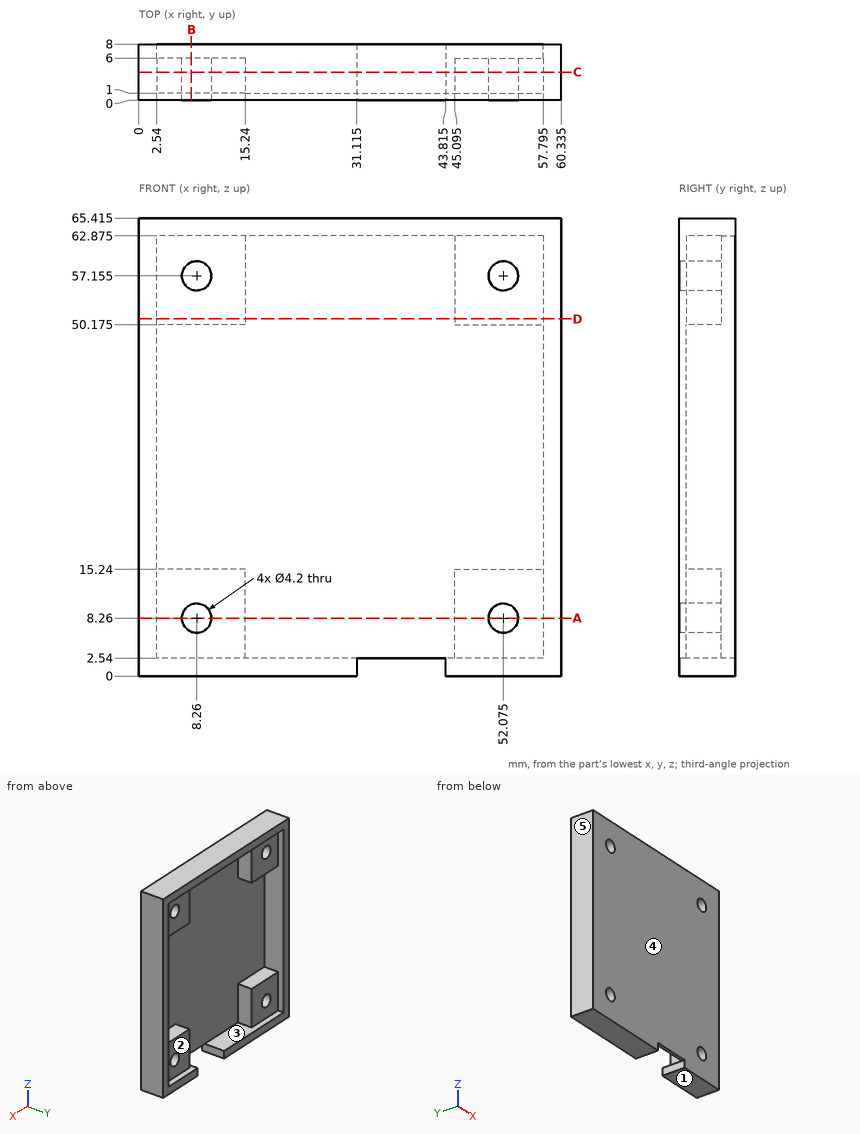
The figure shows three views and two pictorial views of one solid part (mm, origin at its lowest corner). Answer the questions. A direction names the side the tool comes from. Round coordinates to 2 decimals unless told otherwise and drop trailing zeros. Write each loop counter-clockwise with the first axis right and the second up, starting at its lowest first coordinate (ties: lowest second). Pieces come first, ordered by that corner, then holes. Notation, with made-up numbers: (-24.5, 6.5) - (9.5, 6.5) arc R20 ccw to (9.5, 37.5) - close; hole circle Ø3 at (58, -4). An arc over 180 degrees is marked (long way). Use one line per item in the form item = value. Start each with the question number.
Item 1: A cutting plane is placed at A-A (z = 8.26). Write down the section's boundary in (x, y) (3 decimals), plus the area to 3 significant figures.
Item 2: A cutting plane is placed at D-D (z = 51). Write down the section's boundary in (x, y) (3 decimals), plus the area to 3 significant figures.
Item 3: Determine the mould class of the marked faces 3, 4 and 5 for opening direction X: +X half, -X half, draft (parallel to the pull), parting line (faces both ways), or undercut.
Item 4: Flat-ended cylindrical pins translate along their axes: pin 1 Ø4 at (x, z) = (8.26, 57.155) entering from -Y; pin 2 Ø2 at (x, y) = (42.5, 6) entering from -Z (3 decimals); pin 3 Ø4 at (x, z) = (50, 12) entering from +Y. Find the tip coordinate at first contact, or state that the pin passes through.
Item 5: A tool of negligible diameter and unlimited length cuts with its end or side. For the marked faces 1 and 2, from which of +Z, -Z, +X, -X, +Y, -Y can it reach the whole face along a straight path? Write none if from no direction.
Item 6: A cutting plane is placed at C-C (y = 4). Write down the section's boundary in (x, z) (3 decimals), plus the area to 3 significant figures.
Item 7: A cutting plane is placed at B-B (x = 7.5). Write down the section's boundary in (y, z) (3 decimals), plus the area to 3 significant figures.
Item 8: Find the intervals of material crossed by line 1 (Z direction, x = 8.26, y = 3.4) (3 decimals); line 2 (X direction, y = 0.75, z = 8) (3 decimals); line 3 (Z direction, x = 4, y = 2.5) (3 decimals), in increasing order. Write a range as [from, to].
The answers:
q1.outline = (0, 0) - (6.16, 0) - (6.16, 6) - (2.54, 6) - (2.54, 8) - (0, 8) - close; (10.36, 0) - (49.975, 0) - (49.975, 6) - (45.095, 6) - (45.095, 1) - (15.24, 1) - (15.24, 6) - (10.36, 6) - close; (54.175, 0) - (60.335, 0) - (60.335, 8) - (57.795, 8) - (57.795, 6) - (54.175, 6) - close
q1.area = 172 mm^2
q2.outline = (0, 0) - (60.335, 0) - (60.335, 8) - (57.795, 8) - (57.795, 6) - (45.095, 6) - (45.095, 1) - (15.24, 1) - (15.24, 6) - (2.54, 6) - (2.54, 8) - (0, 8) - close
q2.area = 223 mm^2
q3.face_3 = undercut
q3.face_4 = draft
q3.face_5 = -X half
q4.pin_1 = through
q4.pin_2 = 62.875
q4.pin_3 = 6
q5.face_1 = -Z, +X, -X, +Y, -Y
q5.face_2 = +Y
q6.outline = (0, 0) - (31.115, 0) - (31.115, 2.54) - (15.24, 2.54) - (15.24, 15.24) - (2.54, 15.24) - (2.54, 50.175) - (15.24, 50.175) - (15.24, 62.875) - (45.095, 62.875) - (45.095, 50.175) - (57.795, 50.175) - (57.795, 15.24) - (45.095, 15.24) - (45.095, 2.54) - (43.815, 2.54) - (43.815, 0) - (60.335, 0) - (60.335, 65.415) - (0, 65.415) - close; hole circle Ø4.2 at (8.26, 8.26); hole circle Ø4.2 at (8.26, 57.155); hole circle Ø4.2 at (52.075, 8.26); hole circle Ø4.2 at (52.075, 57.155)
q6.area = 1,170 mm^2
q7.outline = (0, 0) - (8, 0) - (8, 2.54) - (6, 2.54) - (6, 6.302) - (0, 6.302) - close; (0, 10.218) - (6, 10.218) - (6, 15.24) - (1, 15.24) - (1, 50.175) - (6, 50.175) - (6, 55.197) - (0, 55.197) - close; (0, 59.113) - (6, 59.113) - (6, 62.875) - (8, 62.875) - (8, 65.415) - (0, 65.415) - close
q7.area = 181 mm^2
q8.line_1 = [0, 6.16], [10.36, 15.24], [50.175, 55.055], [59.255, 65.415]
q8.line_2 = [0, 6.176], [10.344, 49.991], [54.159, 60.335]
q8.line_3 = [0, 15.24], [50.175, 65.415]
